Part model, mm, in its own coordinate system. Coordinates: 2 decimals unless noted, no trailing zeros. Loops run counter-clockwise (first coordinate to the right, second up) from the corner with the lowest first, then second, coordinate; pieces in that order, holes last. Notation, with made-up numbers: (-27, 72) - (-4, 72) arc R14 cw to (-4, 79) - close; hole circle Ø10 at (59, 72.5). An arc over 180 degrees is marked (long way). Use a Markdown table: item, result. Add a question column.
1) Probe probe 1 along Z at (x, y) = (0, 12.5); probe 2 along X at (y, z) = (15, 510); probe 3 along X at (y, z) = (7, -510). List the from-to ranges inside material, lowest first. Write a range as [from, to].
2) Drop flat-ended pins along their axis: P1, Ø1.5, axis at y = 9.5, z = -48.5, coming from the -X side; P2, Ø3, axis at x = -1.5, z = 509.5, coming from the +Y side; P3, Ø2.5, axis at x = 0, z = 521, coming from the -Y side; P4, Ø10.5, axis at x = 0.5, z = -512, coming from the +Y side. Give the stop position or say it passes through.
3) Band-saw the part on A-A (z = -93.5). Give the cut face in (x, y), plus the area to 3 significant figures.
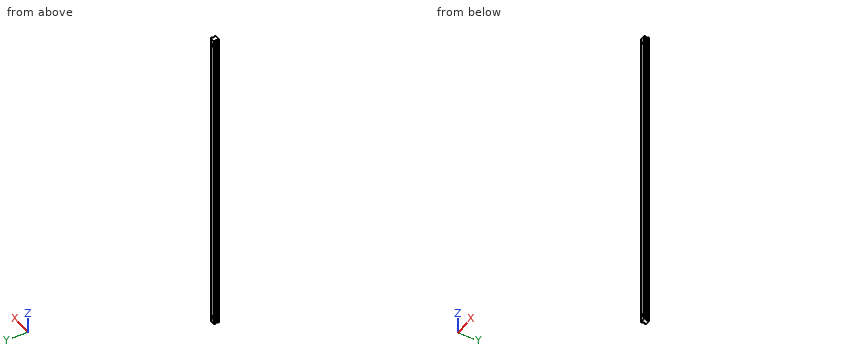
Autodesk Inventor part; units mm, degrees
ref_plane "YZ Plane" through (0, 0, 0) normal (1, 0, 0) x (0, 1, 0)
ref_plane "XZ Plane" through (0, 0, 0) normal (0, 1, 0) x (-1, 0, 0)
ref_plane "XY Plane" through (0, 0, 0) normal (0, 0, 1) x (1, 0, 0)
sketch "Sketch4" plane through (0, 0, 0) normal (0, 0, 1) x (1, 0, 0)
  line L0 (10, 4.0001) -> (10, 1)
  line L1 (6.55, 7.45) -> (10, 4.0001)
  line L2 (6.55, 10.3792) -> (6.55, 7.45)
  line L3 (7.7659, 11.5951) -> (6.55, 10.3792)
  arc A0 (9.4852, 13.3144) -> (7.7659, 11.5951) centre (9.8015, 11.2788) ccw
  line L4 (10, 13.8292) -> (9.4852, 13.3144)
  line L5 (10, 15.16) -> (10, 13.8292)
  line L6 (9.4727, 15.6874) -> (10, 15.16)
  arc A1 (7.7679, 17.3921) -> (9.4727, 15.6874) centre (9.8015, 17.7209) ccw
  line L7 (7.16, 18) -> (7.7679, 17.3921)
  line L8 (-7.16, 18) -> (7.16, 18)
  line L9 (-7.7679, 17.3921) -> (-7.16, 18)
  arc A2 (-9.4727, 15.6874) -> (-7.7679, 17.3921) centre (-9.8015, 17.7209) ccw
  line L10 (-10, 15.16) -> (-9.4727, 15.6874)
  line L11 (-10, 13.8292) -> (-10, 15.16)
  line L12 (-9.4852, 13.3144) -> (-10, 13.8292)
  arc A3 (-7.7659, 11.5951) -> (-9.4852, 13.3144) centre (-9.8015, 11.2788) ccw
  line L13 (-6.55, 10.3792) -> (-7.7659, 11.5951)
  line L14 (-6.55, 7.45) -> (-6.55, 10.3792)
  line L15 (-10, 4.0001) -> (-6.55, 7.45)
  line L16 (-10, 1) -> (-10, 4.0001)
  line L17 (-9, 0) -> (-10, 1)
  line L18 (-3, 0) -> (-9, 0)
  line L19 (-2.5, 0.5) -> (-3, 0)
  line L20 (2.5, 0.5) -> (-2.5, 0.5)
  line L21 (3, 0) -> (2.5, 0.5)
  line L22 (9, 0) -> (3, 0)
  line L23 (10, 1) -> (9, 0)
  point P0 (0, 0)
  point P1 (0, 0)
extrude "Extrusion4" add sketch "Sketch4" along normal mid plane 1060
sketch "Sketch5" plane through (-7.16, 18, 530) normal (0, 1, 0) x (1, 0, 0)
  line L0 (0, 0) -> (14.3201, 0)
  line L1 (0, 1060) -> (0, 0)
  line L2 (7.16, 0) -> (7.16, 20)
  point P0 (7.16, 530)
  dimension "d8" = 20
hole "Hole1" at (0, 18, 510) direction (0, -1, 0) diameter 6 end through all counterbore diameter 9.5 counterbore depth 8.5
pattern_linear "Rectangular Pattern1" count 2 spacing 1020 along (0, 0, -1) of "Hole1"
equation "\"d6\" = L"
equation "\"d8\" = testa"
equation "\"d18\" = passo"
equation "\"passo\" = 1020"
equation "\"testa\" = 20"
properties part number "HSR20-xxxx-01" material "Steel"
Answer block:
| question | item | result |
|---|---|---|
| 1 | probe 1 | [-530, -514.75], [-505.25, 505.25], [514.75, 530] |
| 1 | probe 2 | [-10, -4.75], [4.75, 10] |
| 1 | probe 3 | [-7, -3], [3, 7] |
| 2 | P1 | x = -6.55 |
| 2 | P2 | y = 9.5 |
| 2 | P3 | y = 0.5 |
| 2 | P4 | y = 18 |
| 3 | outline | (-10, 1) - (-9, 0) - (-3, 0) - (-2.5, 0.5) - (2.5, 0.5) - (3, 0) - (9, 0) - (10, 1) - (10, 4) - (6.55, 7.45) - (6.55, 10.38) - (7.77, 11.6) arc R2.06 cw to (9.49, 13.31) - (10, 13.83) - (10, 15.16) - (9.47, 15.69) arc R2.06 cw to (7.77, 17.39) - (7.16, 18) - (-7.16, 18) - (-7.77, 17.39) arc R2.06 cw to (-9.47, 15.69) - (-10, 15.16) - (-10, 13.83) - (-9.49, 13.31) arc R2.06 cw to (-7.77, 11.6) - (-6.55, 10.38) - (-6.55, 7.45) - (-10, 4) - close |
| 3 | area | 302 mm2 |
